```python
from build123d import *

# Parameters (mm, degrees)
SKETCH_1_W          = 40
SKETCH_1_H          = 150
EXTRUDE_1_DEPTH     = 6
SKETCH_2_R          = 1.9
CUT_EXTRUDE_1_DEPTH = 156.357651888
SKETCH_3_W          = 30
SKETCH_3_H          = 59
CUT_EXTRUDE_2_DEPTH = 156.357651888
SKETCH_4_W          = 35
SKETCH_4_H          = 64
CUT_EXTRUDE_3_DEPTH = 3.5
SKETCH_5_W          = 40
SKETCH_5_H          = 7.078158815
SKETCH_5_H_2        = 7.85
CUT_EXTRUDE_4_DEPTH = 1
FILLET_1_R          = 1


with BuildPart() as part:
    # ｽｹｯﾁ1 → ﾎﾞｽ - 押し出し1 (new body)
    with BuildSketch(Plane.XY):
        with Locations((20, 75)):
            Rectangle(SKETCH_1_W, SKETCH_1_H)
    extrude(amount=EXTRUDE_1_DEPTH)

    # ｽｹｯﾁ2 → ｶｯﾄ - 押し出し1 (cut, through all)
    with BuildSketch(Plane.XY.offset(6)):
        with Locations((36, 146.2)):
            Circle(SKETCH_2_R)
        with Locations((4, 146.2)):
            Circle(SKETCH_2_R)
        with Locations((4, 3.8)):
            Circle(SKETCH_2_R)
        with Locations((36, 3.8)):
            Circle(SKETCH_2_R)
    extrude(amount=-CUT_EXTRUDE_1_DEPTH, mode=Mode.SUBTRACT)

    # ｽｹｯﾁ3 → ｶｯﾄ - 押し出し2 (cut, through all)
    with BuildSketch(Plane.XY.offset(6)):
        with Locations((20, 108.5)):
            Rectangle(SKETCH_3_W, SKETCH_3_H)
        with Locations((20, 41.5)):
            Rectangle(SKETCH_3_W, SKETCH_3_H)
    extrude(amount=-CUT_EXTRUDE_2_DEPTH, mode=Mode.SUBTRACT)

    # ｽｹｯﾁ4 → ｶｯﾄ - 押し出し3 (cut)
    with BuildSketch(Plane.XY.offset(6)):
        with Locations((20, 108.5)):
            Rectangle(SKETCH_4_W, SKETCH_4_H)
        with Locations((20, 41.5)):
            Rectangle(SKETCH_4_W, SKETCH_4_H)
    extrude(amount=-CUT_EXTRUDE_3_DEPTH, mode=Mode.SUBTRACT)

    # ｽｹｯﾁ5 → ｶｯﾄ - 押し出し4 (cut)
    with BuildSketch(Plane.XY.offset(6)):
        with Locations((20, 3.539079408)):
            Rectangle(SKETCH_5_W, SKETCH_5_H)
        with Locations((20, 146.075)):
            Rectangle(SKETCH_5_W, SKETCH_5_H_2)
    extrude(amount=-CUT_EXTRUDE_4_DEPTH, mode=Mode.SUBTRACT)

    # ﾌｨﾚｯﾄ1
    fillet_1_edges = [part.edges().sort_by_distance(p)[0] for p in [
        (35, 138, 1.25),
        (35, 79, 1.25),
        (5, 79, 1.25),
        (5, 138, 1.25),
        (35, 71, 1.25),
        (35, 12, 1.25),
        (5, 12, 1.25),
        (5, 71, 1.25),
        (2.5, 76.5, 4.25),
        (2.5, 140.5, 4.25),
        (37.5, 140.5, 4.25),
        (37.5, 76.5, 4.25),
        (2.5, 9.5, 4.25),
        (2.5, 73.5, 4.25),
        (37.5, 73.5, 4.25),
        (37.5, 9.5, 4.25),
    ]]
    fillet(fillet_1_edges, radius=FILLET_1_R)


solid = part.part
```
Read the model definition and answer for the solid it produces. Units are mm, in the model's axes. A direction names the side the tool comes from. Coordinates: 2 decimals unless noted, no trailing zeros. Loops run counter-clockwise (first coordinate to the right, second up) from the corner with the lowest first, then second, coordinate; pieces in that order, holes last. Notation, with made-up numbers: (-14.75, 2) - (14.25, 2) arc R12 ccw to (14.25, 6) - close; hole circle Ø8 at (-2.75, 6). An arc over 180 degrees is marked (long way). Answer in a Markdown table with one row per item.
1. Given pin 1 (17.5 mm diameter, centred on x = 28, y = 123.5, fed in from +Z); pin 2 (5 mm diameter, centred on x = 4, y = 146.2, fed in from -Z); pin 3 (2.5 mm diameter, centred on x = 22.5, y = 147, fed in from +Z), each flat-ended and moving along its own axis, determine where each tip first touches the part or whether it passes through.
Conclusion:
| item | result |
|---|---|
| pin 1 | stops at z = 2.5 |
| pin 2 | stops at z = 0 |
| pin 3 | stops at z = 5 |
2. Find section A-A, the plane x = 22. Write down the section's boundary in (y, z).
Conclusion:
| item | result |
|---|---|
| outline | (0, 0) - (12, 0) - (12, 2.5) - (9.5, 2.5) - (9.5, 6) - (7.08, 6) - (7.08, 5) - (0, 5) - close; (71, 0) - (79, 0) - (79, 2.5) - (76.5, 2.5) - (76.5, 6) - (73.5, 6) - (73.5, 2.5) - (71, 2.5) - close; (138, 0) - (150, 0) - (150, 5) - (142.15, 5) - (142.15, 6) - (140.5, 6) - (140.5, 2.5) - (138, 2.5) - close |
3. Which of the six approach directions +Z, -Z, +X, -X, +Y, -Y give full straight-line access (tool end or side, diameter ignored) to faces 1 (the face through (2.5, 108, 4)), 2 (the face through (35, 41, 1)), 3 (the face through (20, 146, 5)), 4 (the face through (20, 4, 5))?
Conclusion:
| item | result |
|---|---|
| face 1 | +Z |
| face 2 | +Z, -Z |
| face 3 | +Z, +X, -X, +Y |
| face 4 | +Z, +X, -X, -Y |
4. Find section C-C, the plane y = 146.2. Write down the section's boundary in (x, z).
Conclusion:
| item | result |
|---|---|
| outline | (0, 0) - (2.1, 0) - (2.1, 5) - (0, 5) - close; (5.9, 0) - (34.1, 0) - (34.1, 5) - (5.9, 5) - close; (37.9, 0) - (40, 0) - (40, 5) - (37.9, 5) - close |
5. Straight lines are drawn through the part: line 1 (Y direction, x = 36, z = 1.05); line 2 (Y direction, x = 4, z = 3.95); line 3 (Y direction, x = 18, z = 3.4). For each, find the intervals that lie inside material, in ascending order.
Conclusion:
| item | result |
|---|---|
| line 1 | y = 0 to 1.9, 5.7 to 144.3, 148.1 to 150 |
| line 2 | y = 0 to 1.9, 5.7 to 9.5, 73.5 to 76.5, 140.5 to 144.3, 148.1 to 150 |
| line 3 | y = 0 to 9.5, 73.5 to 76.5, 140.5 to 150 |
6. Find section B-B, the plane y = 93. Write down the section's boundary in (x, z).
Conclusion:
| item | result |
|---|---|
| outline | (0, 0) - (5, 0) - (5, 2.5) - (2.5, 2.5) - (2.5, 6) - (0, 6) - close; (35, 0) - (40, 0) - (40, 6) - (37.5, 6) - (37.5, 2.5) - (35, 2.5) - close |
7. Determine the mould class of faces 5 (the face through (40, 74, 3)), 6 (the face through (20, 0, 2)), 7 (the face through (35, 108, 1)), 8 (the face through (0, 74, 3)) for opening direction X: +X half, -X half, draft (parallel to the pull), parting line (faces both ways), or undercut.
Conclusion:
| item | result |
|---|---|
| face 5 | +X half |
| face 6 | draft |
| face 7 | undercut |
| face 8 | -X half |
